Build history of the part. All positions in model axes, mm. Face numbers are marked on the shaded views. Round coordinates to 2 decimals unless told otherwise and drop trailing zeros. Loops run counter-clockwise (first coordinate to the right, second up) from the corner with the lowest first, then second, coordinate; pieces in that order, holes last. Notation, with made-up numbers: (84, 50) - (118, 50) arc R10 ccw to (118, 56) - close; hole circle Ø8 at (-39.75, -29.5). An arc over 180 degrees is marked (long way). Use one line per item in the form item = value. Start each with the question number.
Q1. Pin check, flat tips, straight feed: pin 1 (17 mm diameter, centred on y = 0.5, z = -26, fed in from +X); pin 2 (6 mm diameter, centred on x = -35.5, y = 15.5, fed in from -Z); pin 3 (12 mm diameter, centred on x = -38, z = -7.5, fed in from +Y). Stop position of each tip, or through.
Q2. Saw through at B-B (y = 0). Give the cut face in (x, z), then the cut area to 3 significant figures.
Q3. Mould opens along Z. For the marked faces 1, 2 and 3 say: released by +Z, released by -Z, zero draft, split by the parting line, or undercut.
Q4. Saw through at D-D (y = 17.5). Give the cut face in (x, z), then the cut area to 3 significant figures.
Q5. Saw through at C-C (z = -27). Give the cut face in (x, y).
Q6. Saw through at A-A (x = -11). Give the cut face in (y, z).
Q7. Drill centre lines: line 1 (Y direction, x = -26, z = -1.5); line 2 (Z direction, x = -64, y = 0); line 3 (X direction, y = 4.5, z = -12). Where is each one in solid material? Low to high.
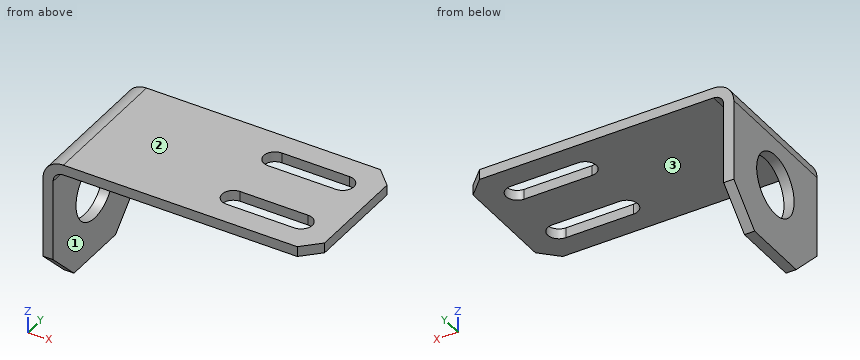
```python
from build123d import *

# Parameters (mm, degrees)
F1_DEPTH = 20
F2_R     = 9
F3_DEPTH = 4
F4_SIZE  = 10
F6_DEPTH = 3
F7_SIZE  = 5


with BuildPart() as f1:
    # F0 (on Front) → F1 (new body, symmetric)
    with BuildSketch(Plane.XZ):
        with BuildLine():
            Line((0, -3), (0, 0))
            Line((0, 0), (-74, 0))
            ThreePointArc((-74, 0), (-78.242641, -1.757359), (-80, -6))
            Line((-80, -6), (-80, -40))
            Line((-80, -40), (-77, -40))
            Line((-77, -40), (-77, -6))
            ThreePointArc((-77, -6), (-76.12132, -3.87868), (-74, -3))
            Line((-74, -3), (0, -3))
        make_face()
    extrude(amount=F1_DEPTH, both=True)

    # F2 (on face) → F3 (cut)
    with BuildSketch(Plane(origin=(-80, 0, 0), x_dir=(0, -1, 0), z_dir=(-1, 0, 0))):
        with Locations((0, -20)):
            Circle(F2_R)
    extrude(amount=-F3_DEPTH, mode=Mode.SUBTRACT)

    # F4
    f4_edges = [f1.edges().sort_by_distance(p)[0] for p in [
        (-78.5, -20, -40),
        (-78.5, 20, -40),
    ]]
    chamfer(f4_edges, length=F4_SIZE)

    # F5 (on face) → F6 (cut)
    with BuildSketch(Plane.XY):
        with BuildLine():
            Line((-10, -6.7), (-30, -6.7))
            ThreePointArc((-30, -6.7), (-33.3, -10), (-30, -13.3))
            Line((-30, -13.3), (-10, -13.3))
            ThreePointArc((-10, -13.3), (-6.7, -10), (-10, -6.7))
        make_face()
        with BuildLine():
            ThreePointArc((-30, 13.3), (-33.3, 10), (-30, 6.7))
            Line((-30, 6.7), (-10, 6.7))
            ThreePointArc((-10, 6.7), (-6.7, 10), (-10, 13.3))
            Line((-10, 13.3), (-30, 13.3))
        make_face()
    extrude(amount=-F6_DEPTH, mode=Mode.SUBTRACT)

    # F7
    f7_edges = [f1.edges().sort_by_distance(p)[0] for p in [
        (0, -20, -1.5),
        (0, 20, -1.5),
    ]]
    chamfer(f7_edges, length=F7_SIZE)


solid = f1.part
```
Report:
q1.pin_1 = -77
q1.pin_2 = -3
q1.pin_3 = 20
q2.outline = (-80, -40) - (-77, -40) - (-77, -29) - (-80, -29) - close; (-80, -11) - (-77, -11) - (-77, -6) arc R3 cw to (-74, -3) - (0, -3) - (0, 0) - (-74, 0) arc R6 ccw to (-80, -6) - close
q2.area = 291 mm²
q3.face_1 = zero draft
q3.face_2 = released by +Z
q3.face_3 = released by -Z
q4.outline = (-80, -32.5) - (-77, -32.5) - (-77, -6) arc R3 cw to (-74, -3) - (-2.5, -3) - (-2.5, 0) - (-74, 0) arc R6 ccw to (-80, -6) - close
q4.area = 315 mm²
q5.outline = (-80, -20) - (-77, -20) - (-77, -5.66) - (-80, -5.66) - close; (-80, 5.66) - (-77, 5.66) - (-77, 20) - (-80, 20) - close
q6.outline = (-20, -3) - (-13.3, -3) - (-13.3, 0) - (-20, 0) - close; (-6.7, -3) - (6.7, -3) - (6.7, 0) - (-6.7, 0) - close; (13.3, -3) - (20, -3) - (20, 0) - (13.3, 0) - close
q7.line_1 = -20 to -13.3, -6.7 to 6.7, 13.3 to 20
q7.line_2 = -3 to 0
q7.line_3 = -80 to -77
